from build123d import *

# Parameters (mm, degrees)
BOSS_EXTRUDE1_DEPTH         = 6
TAP_DRILL_FOR_M6X1_0_TAP1_D = 5


with BuildPart() as part:
    # Sketch2 → Boss-Extrude1 (new, symmetric)
    with BuildSketch(Plane.XY):
        Polygon((-57.7, 90), (57.7, 90), (57.7, 48.5), (35, 48.5), (35, -48.5), (57.7, -48.5), (57.7, -97.0125), (-57.7, -97.0125), (-57.7, -48.5), (-35, -48.5), (-35, 48.5), (-57.7, 48.5), align=None)
    extrude(amount=BOSS_EXTRUDE1_DEPTH, both=True)

    # Tap Drill for M6x1.0 Tap1 (through all)
    with Locations(Plane(origin=(0, 0, -6), x_dir=(-1, 0, 0), z_dir=(0, 0, -1))):
        with Locations((-17.5, 5), (27.5, 5), (27.5, -7), (-17.5, -7)):
            Hole(TAP_DRILL_FOR_M6X1_0_TAP1_D / 2)


solid = part.part
Read the model definition and answer for the solid it produces. Units are mm, in the model's axes. A direction names the side the tool comes from. Give positions to 0.01 mm unless a question says otherwise; leave off trailing zeros. Write each loop counter-clockwise with the first axis right and the second up, starting at its lowest first coordinate (ties: lowest second). Pieces come first, ordered by that corner, then holes. Notation, with made-up numbers: M 24,-38.75 L 69,-38.75 A28 ccw 69,-0.75 Z; hole C 61.5,85 d11. An arc over 180 degrees is marked long. One line per item, written item: value. Start each with the question number.
(1) Find the intervals of material crossed by line 1 (Y direction, x = 17.5, z = -2.75); line 2 (Y direction, x = 38.5, z = 5); line 3 (X direction, y = -21.5, z = 0), in increasing order.
(2) Flat-ended cylindrical pins translate along their axes: pin 1 Ø4 at (y, z) = (41, -0.5) entering from -X; pin 2 Ø2 at (y, z) = (22, -1.5) entering from +X. Find the tip coordinate at first contact, or state that the pin passes through.
(3) A tool of negligible diameter and unlimited length cuts with its end or side. For faces 5 (the flat face through (1, -2, -6)), 6 (the flat face through (35, 1, 0)), 7 (the flat face through (-46, 48.5, 0)), from which of +Z, -Z, +X, -X, +Y, -Y can it reach the whole face along a straight path? Write none if from no direction.
(4) Find section D-D (y = 25). Determine the outline of the cut face in (x, z).
(5) Find section C-C (y = 5). Determine the outline of the cut face in (x, z).
(6) Find section B-B (z = -3.5). Determine the outline of the cut face in (x, y).
(7) Determine the mould class of faces 1 (the flat face through (-1, 90, 0)), 2 (the flat face through (1, -97.012, 0)), 3 (the flat face through (46, -48.5, 0)), 4 (the flat face through (57.7, 70, 0)) for opening direction Y: pulls with the +Y half, pulls with the -Y half, needs draft (parallel to the pull), parting line crosses it, or undercut.
(8) Find section A-A (x = 17.5). Determine the outline of the cut face in (y, z).
Results below:
1. line 1: y = -97.01 to -9.5, -4.5 to 2.5, 7.5 to 90
1. line 2: y = -97.01 to -48.5, 48.5 to 90
1. line 3: x = -35 to 35
2. pin 1: stops at x = -35
2. pin 2: stops at x = 35
3. face 5: -Z, +X, -X, +Y, -Y
3. face 6: +Z, -Z, +X
3. face 7: +Z, -Z, -X
4. outline: M -35,-6 L 35,-6 L 35,6 L -35,6 Z
5. outline: M -35,-6 L -30,-6 L -30,6 L -35,6 Z; M -25,-6 L 15,-6 L 15,6 L -25,6 Z; M 20,-6 L 35,-6 L 35,6 L 20,6 Z
6. outline: M -57.7,-97.01 L 57.7,-97.01 L 57.7,-48.5 L 35,-48.5 L 35,48.5 L 57.7,48.5 L 57.7,90 L -57.7,90 L -57.7,48.5 L -35,48.5 L -35,-48.5 L -57.7,-48.5 Z; hole C -27.5,-7 d5; hole C -27.5,5 d5; hole C 17.5,-7 d5; hole C 17.5,5 d5
7. face 1: pulls with the +Y half
7. face 2: pulls with the -Y half
7. face 3: undercut
7. face 4: needs draft
8. outline: M -97.01,-6 L -9.5,-6 L -9.5,6 L -97.01,6 Z; M -4.5,-6 L 2.5,-6 L 2.5,6 L -4.5,6 Z; M 7.5,-6 L 90,-6 L 90,6 L 7.5,6 Z
